Autodesk Inventor part; units mm, degrees
ref_plane "YZ Plane" through (0, 0, 0) normal (1, 0, 0) x (0, 1, 0)
ref_plane "XZ Plane" through (0, 0, 0) normal (0, 1, 0) x (-1, 0, 0)
ref_plane "XY Plane" through (0, 0, 0) normal (0, 0, 1) x (1, 0, 0)
sketch "Esboço1" plane through (0, 0, 0) normal (1, 0, 0) x (0, 1, 0)
  line L0 (0, 0) -> (0, -572.55)
  line L1 (0, 0) -> (7.5, 0)
  line L2 (7.5, 0) -> (7.5, -572.55)
  line L3 (7.5, -572.55) -> (0, -572.55)
  line L4 (0, -572.55) -> (0, 0)
  line L5 (7.5, -15) -> (25.4, -15)
  line L6 (25.4, -15) -> (25.4, -557.55)
  line L7 (25.4, -557.55) -> (7.5, -557.55)
  line L8 (7.5, -557.55) -> (7.5, -15)
  point P0 (3.75, 0)
  point P1 (3.75, -572.55)
  point P2 (0, -545.49)
  point P3 (7.5, -557.55)
  dimension "d0" = 572.55
  dimension "d1" = 7.5
  dimension "d2" = 25.4
  dimension "d3" = 15
  dimension "d4" = 15
revolve "Revolução1" add sketch "Esboço1" angle 360 about axis through (0, 0, -572.55) along (0, 0, 1)
sketch "Esboço2" plane through (0, 0, -15) normal (0, 0, 1) x (1, 0, 0)
  circle A0 centre (0, 0) radius 7.5
  circle A1 centre (0, 0) radius 25.4
  circle A2 centre (0, 0) radius 7.5
  line L0 (0, 0) -> (0, 25.4)
  line L1 (0, 0) -> (-25.4, 0)
  line L2 (0, 0) -> (0, -25.4)
  line L3 (0, 0) -> (25.4, 0)
  line L4 (0, 0) -> (17.9605, 17.9605)
  line L5 (0, 0) -> (9.7202, 23.4665)
  line L6 (0, 0) -> (23.4665, 9.7202)
  line L7 (0, 0) -> (-17.9605, 17.9605)
  line L8 (0, 0) -> (-9.7202, 23.4665)
  line L9 (0, 0) -> (-23.4665, 9.7202)
  line L10 (0, 0) -> (17.9605, -17.9605)
  line L11 (0, 0) -> (9.7202, -23.4665)
  line L12 (0, 0) -> (23.4665, -9.7202)
  line L13 (0, 0) -> (-9.7202, -23.4665)
  line L14 (0, 0) -> (-17.9605, -17.9605)
  line L15 (0, 0) -> (-23.4665, -9.7202)
  circle A3 centre (0, 0) radius 19.4
  point P0 (0, 0)
  point P1 (-17.9233, 7.4241)
  point P2 (-13.7179, 13.7179)
  point P3 (-17.9233, -7.4241)
  point P4 (-19.4, 0)
  point P5 (-7.4241, -17.9233)
  point P6 (-13.7179, -13.7179)
  point P7 (7.4241, -17.9233)
  point P8 (0, -19.4)
  point P9 (17.9233, -7.4241)
  point P10 (13.7179, -13.7179)
  point P11 (17.9233, 7.4241)
  point P12 (19.4, 0)
  point P13 (7.4241, 17.9233)
  point P14 (13.7179, 13.7179)
  point P15 (-7.4241, 17.9233)
  point P16 (0, 19.4)
  dimension "d8" = 22.5
  dimension "d9" = 22.5
  dimension "d10" = 45
  dimension "d11" = 6
extrude "Extrusão1" cut sketch "Esboço2" against normal up to surface (542.55 mm away) contours A3 L6 A1 L3 | L12 A1 L10 A3 | A3 L5 A1 L4 | A3 L8 A1 L0 | A3 L15 A1 L1 | A3 L11 A1 L2 | A3 L9 A1 L7 | L13 A1 L14 A3
fillet "Arredondamento1" radius 3 31 edges at (7.4241, 17.9233, -286.275) (13.7179, 13.7179, -286.275) (17.9605, 17.9605, -286.275) (9.7202, 23.4665, -286.275) (0, 25.4, -286.275) (0, 19.4, -286.275) (-9.7202, 23.4665, -286.275) (-7.4241, 17.9233, -286.275) (-23.4665, 9.7202, -286.275) (-17.9605, 17.9605, -286.275) (-17.9233, 7.4241, -286.275) (-13.7179, 13.7179, -286.275) (19.4, 0, -286.275) (17.9233, 7.4241, -286.275) (23.4665, 9.7202, -286.275) (25.4, 0, -286.275) (23.4665, -9.7202, -286.275) (17.9233, -7.4241, -286.275) (17.9605, -17.9605, -286.275) (13.7179, -13.7179, -286.275) (7.4241, -17.9233, -286.275) (9.7202, -23.4665, -286.275) (0, -19.4, -286.275) (-9.7202, -23.4665, -286.275) (-7.4241, -17.9233, -286.275) (-13.7179, -13.7179, -286.275) (-23.4665, -9.7202, -286.275) (-17.9605, -17.9605, -286.275) (-19.4, 0, -286.275) (-25.4, 0, -286.275) (0, -25.4, -286.275)
equation "\"d9\" = d8"
properties part number "Coletor - Intake"
The model under review builds one solid part; all positions refer to its coordinate system, in mm. A direction names the side the tool comes from. Round coordinates to 2 decimals unless told otherwise and drop trailing zeros. Answer as CSV lines item,"result". Start each with the question number.
Item 1: Wall thickness on line 1 (Z direction, x = -12.5, y = 10); line 2 (X direction, y = 23, z = -481); line 3 (X direction, y = 16, z = -55.5): over which ranges is each line inside the solid? List them lowest first. Write a range as [from, to].
Item 2: For faces 1 (the face through (0.33, -7.493, -7.605)), 2 (the face through (0, 0, -572.55)), 3 (the face through (0.33, -7.493, -565.155)), list the 3-axis set-ups (+Z, -Z, +X, -X, +Y, -Y) from which the entire face can be reached by the end or side of a thin tool; tool diameter is ignored.
Item 3: Insertion check: P1, Ø1, axis at x = 13, z = -376, coming from the +Y side; P2, Ø10, axis at x = 20, y = 5, coming from the -Z side; P3, Ø2, axis at y = 16, z = -265, coming from the +X side; P4, Ø3, axis at x = -2, y = -3, coming from the +Z side. Each pin has a flat end and moves straight along its axis. Give the tip position at first contact, or say it passes through.
Answer:
1,line 1,"z = [-557.55, -15]"
1,line 2,"x = [0.11, 8.41]"
1,line 3,"x = [-15.96, 10.97], [16.05, 19.58]"
2,face 1,"+Z"
2,face 2,"-Z, +X, -X, +Y, -Y"
2,face 3,"-Z"
3,P1,"stops at y = 15.02"
3,P2,"stops at z = -557.55"
3,P3,"stops at x = 20.5"
3,P4,"stops at z = 0"
